For this review, use the dimensioned drawing (mm, ordinates from the lowest corner) and the shaded views. A direction names the side the tool comes from. Coordinates: 2 decimals unless noted, no trailing zeros. Order: outer loops, then holes, each group sorted by start corner. A loop starts at its lowest first (then second) coordinate and runs counter-clockwise, first axis right, second up. Notation, with made-up numbers: M -26.75,-10.5 L 23.25,-10.5 A26 ccw 23.25,17.5 Z; hole C -20.75,71.25 d10. An arc over 180 degrees is marked long. Answer in a Markdown table with one row per item.
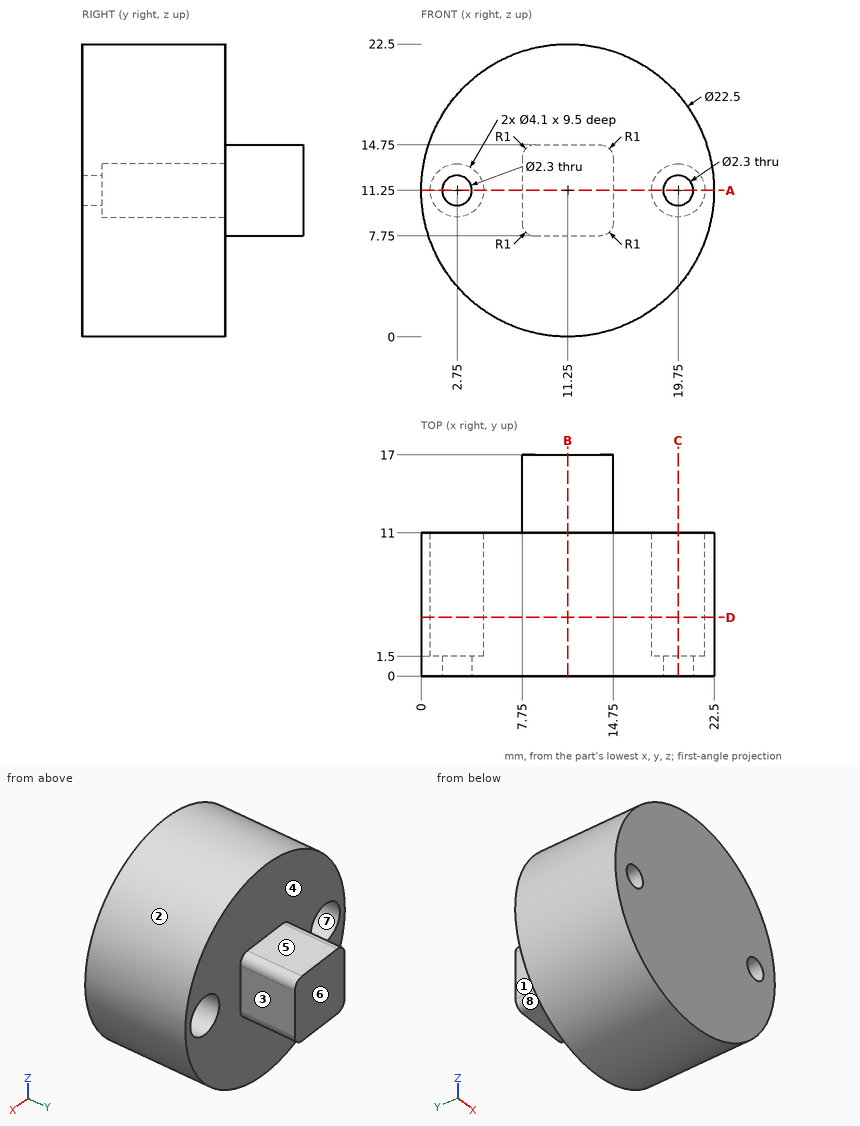
(1) Machinability: for the marked faces 1, 2, 3, 4 and 5, which of the approach directions +Z, -Z, +X, -X, +Y, -Y give a long, thin tool a straight path to every point of the face, cutting with its end or side? Answer none if there is none.
Report:
| item | result |
|---|---|
| face 1 | +Z, -Z, -X, +Y |
| face 2 | +Y, -Y |
| face 3 | +Z, -Z, +X, +Y |
| face 4 | +Y |
| face 5 | +Z, +X, -X, +Y |
(2) Take a section at D-D (y = 4.5). Write out the cut boundary in (x, z).
Report:
| item | result |
|---|---|
| outline | C 11.25,11.25 d22.5; hole C 2.75,11.25 d4.1; hole C 19.75,11.25 d4.1 |
(3) Take a section at B-B (x = 11.25). Write out the cut boundary in (y, z), then the cut area to 4 significant figures.
Report:
| item | result |
|---|---|
| outline | M 0,0 L 11,0 L 11,7.75 L 17,7.75 L 17,14.75 L 11,14.75 L 11,22.5 L 0,22.5 Z |
| area | 289.5 mm^2 |
(4) Take a section at A-A (z = 11.25). Write out the cut boundary in (x, y), then the cut area to 3 significant figures.
Report:
| item | result |
|---|---|
| outline | M 0,0 L 1.6,0 L 1.6,1.5 L 0.7,1.5 L 0.7,11 L 0,11 Z; M 3.9,0 L 18.6,0 L 18.6,1.5 L 17.7,1.5 L 17.7,11 L 14.75,11 L 14.75,17 L 7.75,17 L 7.75,11 L 4.8,11 L 4.8,1.5 L 3.9,1.5 Z; M 20.9,0 L 22.5,0 L 22.5,11 L 21.8,11 L 21.8,1.5 L 20.9,1.5 Z |
| area | 205 mm^2 |
(5) The part is to be moulded in two halves that separate along X. For the marked faces 6, 7 and 8, say which applies: +X half, -X half, draft (parallel to the pull), parting line (faces both ways), or undercut.
Report:
| item | result |
|---|---|
| face 6 | draft |
| face 7 | undercut |
| face 8 | -X half |
(6) Take a section at C-C (x = 19.75). Write out the cut boundary in (y, z).
Report:
| item | result |
|---|---|
| outline | M 0,3.88 L 11,3.88 L 11,9.2 L 1.5,9.2 L 1.5,10.1 L 0,10.1 Z; M 0,12.4 L 1.5,12.4 L 1.5,13.3 L 11,13.3 L 11,18.62 L 0,18.62 Z |
(7) Insertion check: P1, Ø2.5, axis at y = 15, z = 11.5, coming from the -X side; P2, Ø2, axis at x = 19, z = 13, coming from the -Y side; P3, Ø8, axis at x = 15, y = 13, coming from the -Z side; P4, Ø2.5, axis at x = 11, y = 13.5, coming from the -Z side. Each pin has a flat end and moves straight along its axis. Give the tip position at first contact, or say it passes through.
Report:
| item | result |
|---|---|
| P1 | x = 7.75 |
| P2 | y = 0 |
| P3 | z = 0 |
| P4 | z = 7.75 |
(8) To check wall thickness, follow line 1 (X direction, y = 5.5, z = 11.25); line 2 (X direction, y = 0.5, z = 11.25); line 3 (Y direction, x = 2, z = 16.75). State the ranges of each line that lie inside material, in increasing order. Write a range as [from, to].
Report:
| item | result |
|---|---|
| line 1 | [0, 0.7], [4.8, 17.7], [21.8, 22.5] |
| line 2 | [0, 1.6], [3.9, 18.6], [20.9, 22.5] |
| line 3 | [0, 11] |
